The drawing under review shows one solid part. Ordinate dimensions are in mm from its lowest x, y, z. A direction names the side the tool comes from. Round coordinates to 2 decimals unless told otherwise and drop trailing zeros. Loops run counter-clockwise (first coordinate to the right, second up) from the corner with the lowest first, then second, coordinate; pieces in that order, holes last. Notation, with made-up numbers: M 56,69 L 108,69 A25 ccw 108,85 Z; hole C 39,-38.75 d7. An arc over 180 degrees is marked long. Use a Markdown table: item, result.
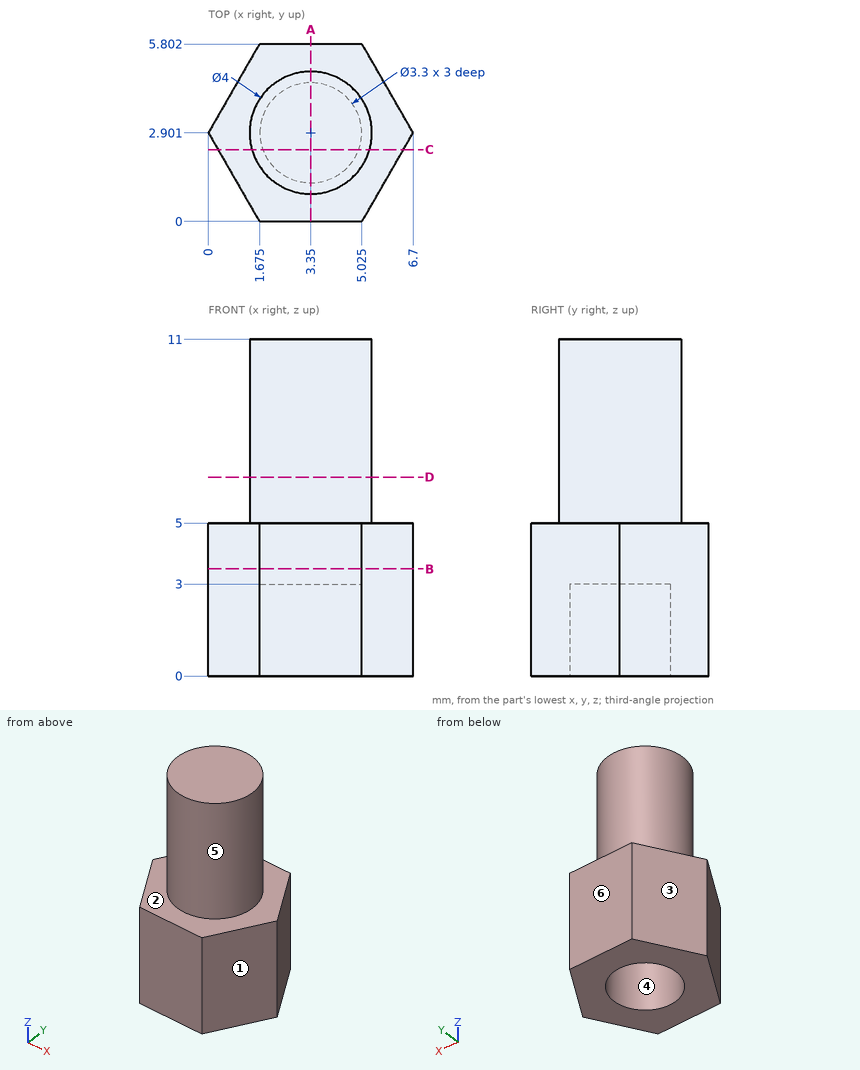
1. The part is to be moulded in two halves that separate along X. For the marked faces 3, 4, 5 and 6, say which applies: pulls with the +X half, pulls with the -X half, needs draft (parallel to the pull), parting line crosses it, or undercut.
Check values:
| item | result |
|---|---|
| face 3 | pulls with the -X half |
| face 4 | undercut |
| face 5 | parting line crosses it |
| face 6 | needs draft |
2. Wall thickness on line 1 along Y through (x, z) = (3.35, 2.4); line 2 along Z through (x, y) = (1.5, 4.95); line 3 along X through (y, z) = (2.85, 10): over which ranges is each line inside the solid? List them lowest first. Write a range as from..to.
Check values:
| item | result |
|---|---|
| line 1 | y = 0..1.25, 4.55..5.8 |
| line 2 | z = 0..5 |
| line 3 | x = 1.35..5.35 |
3. Take a section at C-C on y = 2.35. Give the boundary of the cut face in (x, z) (1 decimal).
Check values:
| item | result |
|---|---|
| outline | M 0.3,0 L 1.8,0 L 1.8,3 L 4.9,3 L 4.9,0 L 6.4,0 L 6.4,5 L 5.3,5 L 5.3,11 L 1.4,11 L 1.4,5 L 0.3,5 Z |
4. Machinability: for the marked faces 1 and 2, which of the approach directions +Z, -Z, +X, -X, +Y, -Y give a long, thin tool a straight path to every point of the face, cutting with its end or side? Answer none if there is none.
Check values:
| item | result |
|---|---|
| face 1 | +Z, -Z, +X, -Y |
| face 2 | +Z |
5. Insertion check: pin 1 (2 mm diameter, centred on y = 0.5, z = 8.5, fed in from -X). The pin has a flat end and moves straight along its axis. Give the tip position at first contact, or say it passes through.
Check values:
| item | result |
|---|---|
| pin 1 | stops at x = 1.92 |
6. Take a section at B-B on z = 3.5. Give the boundary of the cut face in (x, y) (1 decimal).
Check values:
| item | result |
|---|---|
| outline | M 0,2.9 L 1.7,0 L 5,0 L 6.7,2.9 L 5,5.8 L 1.7,5.8 Z |
7. Take a section at D-D on z = 6.5. Give the boundary of the cut face in (x, y), and give its area (3 significant figures).
Check values:
| item | result |
|---|---|
| outline | C 3.35,2.9 d4 |
| area | 12.6 mm² |
8. Take a section at A-A on x = 3.35. Give the boundary of the cut face in (y, z).
Check values:
| item | result |
|---|---|
| outline | M 0,0 L 1.25,0 L 1.25,3 L 4.55,3 L 4.55,0 L 5.8,0 L 5.8,5 L 4.9,5 L 4.9,11 L 0.9,11 L 0.9,5 L 0,5 Z |
